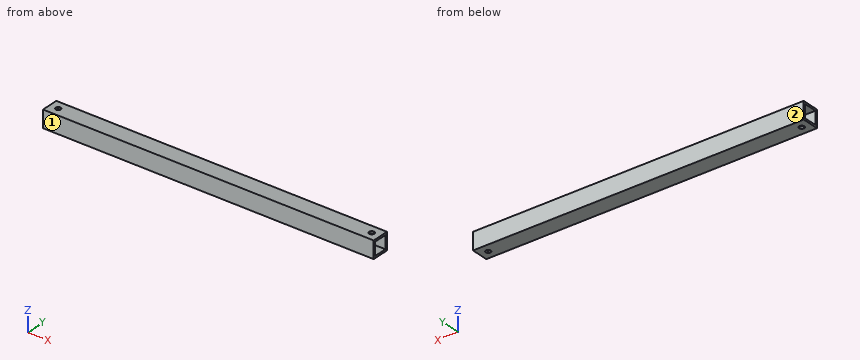
Autodesk Inventor part; units mm, degrees
ref_plane "YZ Plane" through (0, 0, 0) normal (1, 0, 0) x (0, 1, 0)
ref_plane "XZ Plane" through (0, 0, 0) normal (0, 1, 0) x (-1, 0, 0)
ref_plane "XY Plane" through (0, 0, 0) normal (0, 0, 1) x (1, 0, 0)
sketch "スケッチ2" plane through (0, 0, 0) normal (0, 0, 1) x (1, 0, 0)
  line L0 (0, 0) -> (148.4693, 71.9851)
  line L1 (148.4693, 71.9851) -> (183.3712, 0)
  line L2 (0, 0) -> (183.3712, 0)
  line L3 (-5, -5) -> (188.3712, -5)
  line L4 (188.3712, -5) -> (188.3712, 5)
  line L5 (188.3712, 5) -> (-5, 5)
  line L6 (-5, 5) -> (-5, -5)
  dimension "d3" = 165
  dimension "d4" = 80
  dimension "d5" = 10
  dimension "d6" = 5
  dimension "d7" = 5
extrude "押し出し1" add sketch "スケッチ2" along normal blind 10 contours L2 L1 L5 L4 L3 L6 L0 | L0 L5 L1 L2
sketch "スケッチ3" plane through (188.3712, -5, 0) normal (1, 0, 0) x (0, 0, -1)
  line L0 (0, 0) -> (0, 10)
  line L1 (0, 10) -> (-10, 10)
  line L2 (-10, 0) -> (-10, 10)
  line L3 (0, 0) -> (-10, 0)
  line L4 (-8.8, 8.8) -> (-1.2, 8.8)
  line L5 (-1.2, 8.8) -> (-1.2, 1.2)
  line L6 (-1.2, 1.2) -> (-8.8, 1.2)
  line L7 (-8.8, 1.2) -> (-8.8, 8.8)
  point P0 (0, 5)
  dimension "d10" = 1.2
extrude "押し出し2" cut sketch "スケッチ3" against normal through all contours L4 L5 L6 L7
hole "穴1" at (0, 0, 0) at (183.3712, 0, 0) direction (0, 0, 1) diameter 3 end through all
properties part number "truss_1010_zegi" material "アルミニウム 6061-AHC"
The model under review builds one solid part; all positions refer to its coordinate system, in mm. Face numbers are marked on the shaded views. Round coordinates to 2 decimals unless told otherwise and drop trailing zeros. Write each loop counter-clockwise with the first axis right and the second up, starting at its lowest first coordinate (ties: lowest second). Pieces come first, ordered by that corner, then holes. Notation, with made-up numbers: M -0.75,56 L 15.25,56 A27 ccw 15.25,95 Z; hole C 57,70.25 d1. An arc over 180 degrees is marked long. Use a Markdown table: item, result. Add a question column.
Q1. The part is to be moulded in two halves that separate along Y. For the marked faces 1 and 2, say which applies: pulls with the +Y half, pulls with the -Y half, needs draft (parallel to the pull), parting line crosses it, or undercut.
Q2. We need section A-A, the plane y = 0. State the section outline as (x, z) points.
Q3. To check wall thickness, follow line 1 (X direction, y = 0, z = 9.35); line 2 (Y direction, x = 179.5, z = 3.25); line 3 (Z direction, x = 116, y = 3). State the ranges of each line that lie inside material, in increasing order.
Q4. We need section B-B, the plane x = 145. State the section outline as (y, z) points.
Q5. We need section C-C, the plane z = 4.5. State the section outline as (x, y) points, plus the area to 3 significant figures.
Findings below:
| question | item | result |
|---|---|---|
| 1 | face 1 | pulls with the -Y half |
| 1 | face 2 | pulls with the +Y half |
| 2 | outline | M -5,0 L -1.5,0 L -1.5,1.2 L -5,1.2 Z; M -5,8.8 L -1.5,8.8 L -1.5,10 L -5,10 Z; M 1.5,0 L 181.87,0 L 181.87,1.2 L 1.5,1.2 Z; M 1.5,8.8 L 181.87,8.8 L 181.87,10 L 1.5,10 Z; M 184.87,0 L 188.37,0 L 188.37,1.2 L 184.87,1.2 Z; M 184.87,8.8 L 188.37,8.8 L 188.37,10 L 184.87,10 Z |
| 3 | line 1 | x = -5 to -1.5, 1.5 to 181.87, 184.87 to 188.37 |
| 3 | line 2 | y = -5 to -3.8, 3.8 to 5 |
| 3 | line 3 | z = 0 to 1.2, 8.8 to 10 |
| 4 | outline | M -5,0 L 5,0 L 5,10 L -5,10 Z; hole M -3.8,1.2 L 3.8,1.2 L 3.8,8.8 L -3.8,8.8 Z |
| 5 | outline | M -5,-5 L 188.37,-5 L 188.37,-3.8 L -5,-3.8 Z; M -5,3.8 L 188.37,3.8 L 188.37,5 L -5,5 Z |
| 5 | area | 464 mm² |
